from build123d import *
from build123d.topology import SkipClean

# Parameters (mm, degrees)
SKETCH_1_R               = 82.5
SKETCH_1_R_2             = 11.5
EXTRUDE_1_DEPTH          = 5
SKETCH_2_R               = 4
SKETCH_2_R_2             = 2.1
EXTRUDE_2_DEPTH          = 15
EXTRUDE_START            = 5
SKETCH_3_R               = 34
SKETCH_3_R_2             = 11.5
EXTRUDE_3_DEPTH          = 5
CUT_EXTRUDE_1_DEPTH      = 118.63290356
CUT_EXTRUDE_1_DEPTH_BACK = 10
SKETCH_4_R               = 82.5
EXTRUDE_4_DEPTH          = 5
SKETCH_6_R               = 11.5
CUT_EXTRUDE_2_DEPTH      = 109.80791311
SKETCH_7_R               = 34.75
SKETCH_7_R_2             = 11.5
EXTRUDE_5_DEPTH          = 5


with BuildPart() as part:
    # 草圖1 → 填料-伸長1 (new body)
    with BuildSketch(Plane(origin=(0, 0, 0), x_dir=(1, 0, 0), z_dir=(0, 1, 0))):
        with Locations(Location((0, 0, 0), (0, 0, 270))):
            Circle(SKETCH_1_R)
        with Locations(Location((0, 0, 0), (0, 0, 270))):
            Circle(SKETCH_1_R_2, mode=Mode.SUBTRACT)
    extrude(amount=EXTRUDE_1_DEPTH)

    # 草圖2 → 填料-伸長2 (add)
    # profile 1 of 3: a face of its own
    with BuildSketch(Plane(origin=(0, 5, 0), x_dir=(1, 0, 0), z_dir=(0, 1, 0))):
        with Locations(Location((0, 71.25, 0), (0, 0, 270))):
            Circle(SKETCH_2_R)
        with Locations(Location((0, 71.25, 0), (0, 0, 270))):
            Circle(SKETCH_2_R_2, mode=Mode.SUBTRACT)
    # profile 2 of 3: a face of its own
    with BuildSketch(Plane(origin=(0, 5, 0), x_dir=(1, 0, 0), z_dir=(0, 1, 0))):
        with Locations(Location((61.70431002, -35.625, 0), (0, 0, 270))):
            Circle(SKETCH_2_R)
        with Locations(Location((61.70431002, -35.625, 0), (0, 0, 270))):
            Circle(SKETCH_2_R_2, mode=Mode.SUBTRACT)
    # profile 3 of 3: a face of its own
    with BuildSketch(Plane(origin=(0, 5, 0), x_dir=(1, 0, 0), z_dir=(0, 1, 0))):
        with Locations(Location((-61.70431002, -35.625, 0), (0, 0, 270))):
            Circle(SKETCH_2_R)
        with Locations(Location((-61.70431002, -35.625, 0), (0, 0, 270))):
            Circle(SKETCH_2_R_2, mode=Mode.SUBTRACT)
    extrude(amount=EXTRUDE_2_DEPTH)

    # 草圖3 → 填料-伸長3 (add)
    with SkipClean():  # the faces are left unmerged after this step: merging them gives an invalid solid
        with BuildSketch(Plane.XZ.offset(EXTRUDE_START)):
            with Locations(Location((0, 0, 0), (0, 0, 90))):
                Circle(SKETCH_3_R)
            with Locations(Location((0, 0, 0), (0, 0, 270))):
                Circle(SKETCH_3_R_2, mode=Mode.SUBTRACT)
        extrude(amount=-EXTRUDE_3_DEPTH)

    # 草圖4 → 除料-伸長1 (cut, two sides: drawn at the far end of the back side and taken through both)
    with SkipClean():  # the faces are left unmerged after this step: merging them gives an invalid solid
        with BuildSketch(Plane(origin=(0, 5, 0), x_dir=(1, 0, 0), z_dir=(0, 1, 0)).offset(-CUT_EXTRUDE_1_DEPTH_BACK)):
            Circle(SKETCH_4_R)
            with BuildLine():
                ThreePointArc((-34.463200133, -38.269280586), (0, -51.5), (34.463200133, -38.269280586))
                ThreePointArc((34.463200133, -38.269280586), (40.109412614, -35.755030522), (46.155083654, -37.039954818))
                Line((46.155083654, -37.039954818), (57.20431002, -43.419228634))
                ThreePointArc((57.20431002, -43.419228634), (69.498538654, -40.125), (66.20431002, -27.830771366))
                Line((66.20431002, -27.830771366), (55.155083654, -21.451497549))
                ThreePointArc((55.155083654, -21.451497549), (51.019471053, -16.858254994), (50.373769239, -10.711366518))
                ThreePointArc((50.373769239, -10.711366518), (44.600308295, 25.75), (15.910569106, 48.980647104))
                ThreePointArc((15.910569106, 48.980647104), (10.910058438, 52.613285516), (9, 58.491452367))
                Line((9, 58.491452367), (9, 71.25))
                ThreePointArc((9, 71.25), (0, 80.25), (-9, 71.25))
                Line((-9, 71.25), (-9, 58.491452367))
                ThreePointArc((-9, 58.491452367), (-10.910058438, 52.613285516), (-15.910569106, 48.980647104))
                ThreePointArc((-15.910569106, 48.980647104), (-44.600308295, 25.75), (-50.373769239, -10.711366518))
                ThreePointArc((-50.373769239, -10.711366518), (-51.019471053, -16.858254994), (-55.155083654, -21.451497549))
                Line((-55.155083654, -21.451497549), (-66.20431002, -27.830771366))
                ThreePointArc((-66.20431002, -27.830771366), (-69.498538654, -40.125), (-57.20431002, -43.419228634))
                Line((-57.20431002, -43.419228634), (-46.155083654, -37.039954818))
                ThreePointArc((-46.155083654, -37.039954818), (-40.109412614, -35.755030522), (-34.463200133, -38.269280586))
            make_face(mode=Mode.SUBTRACT)
        extrude(amount=CUT_EXTRUDE_1_DEPTH + CUT_EXTRUDE_1_DEPTH_BACK, mode=Mode.SUBTRACT)

    # 草圖5 → 填料-伸長4 (add)
    with BuildSketch(Plane.XZ):
        with BuildLine():
            Line((-46.155083654, 37.039954818), (-57.20431002, 43.419228634))
            ThreePointArc((-57.20431002, 43.419228634), (-69.498538654, 40.125), (-66.20431002, 27.830771366))
            Line((-66.20431002, 27.830771366), (-55.155083654, 21.451497549))
            ThreePointArc((-55.155083654, 21.451497549), (-51.019471053, 16.858254994), (-50.373769239, 10.711366518))
            ThreePointArc((-50.373769239, 10.711366518), (-44.600308295, -25.75), (-15.910569106, -48.980647104))
            ThreePointArc((-15.910569106, -48.980647104), (-10.910058438, -52.613285516), (-9, -58.491452367))
            Line((-9, -58.491452367), (-9, -71.25))
            ThreePointArc((-9, -71.25), (0, -80.25), (9, -71.25))
            Line((9, -71.25), (9, -58.491452367))
            ThreePointArc((9, -58.491452367), (10.910058438, -52.613285516), (15.910569106, -48.980647104))
            ThreePointArc((15.910569106, -48.980647104), (44.600308295, -25.75), (50.373769239, 10.711366518))
            ThreePointArc((50.373769239, 10.711366518), (51.019471053, 16.858254994), (55.155083654, 21.451497549))
            Line((55.155083654, 21.451497549), (66.20431002, 27.830771366))
            ThreePointArc((66.20431002, 27.830771366), (69.498538654, 40.125), (57.20431002, 43.419228634))
            Line((57.20431002, 43.419228634), (46.155083654, 37.039954818))
            ThreePointArc((46.155083654, 37.039954818), (40.109412614, 35.755030522), (34.463200133, 38.269280586))
            ThreePointArc((34.463200133, 38.269280586), (0, 51.5), (-34.463200133, 38.269280586))
            ThreePointArc((-34.463200133, 38.269280586), (-40.109412614, 35.755030522), (-46.155083654, 37.039954818))
        make_face()
    extrude(amount=EXTRUDE_4_DEPTH)

    # 草圖6 → 除料-伸長2 (cut, through all)
    with BuildSketch(Plane(origin=(0, 0, 0), x_dir=(1, 0, 0), z_dir=(0, 1, 0))):
        with Locations(Location((0, 0, 0), (0, 0, 270))):
            Circle(SKETCH_6_R)
    extrude(amount=-CUT_EXTRUDE_2_DEPTH, mode=Mode.SUBTRACT)

    # 草圖7 → 填料-伸長5 (add)
    with SkipClean():  # the faces are left unmerged after this step: merging them gives an invalid solid
        with BuildSketch(Plane.XZ.offset(5)):
            with Locations(Location((0, 0, 0), (0, 0, 270))):
                Circle(SKETCH_7_R)
            with Locations(Location((0, 0, 0), (0, 0, 270))):
                Circle(SKETCH_7_R_2, mode=Mode.SUBTRACT)
        extrude(amount=EXTRUDE_5_DEPTH)
    add(part.part.scale(1), mode=Mode.REPLACE)  # the faces are merged on a copy


solid = part.part
For this review, take the finished solid that the model builds, in its own axes (mm). A direction names the side the tool comes from. Round coordinates to 2 decimals unless told otherwise and drop trailing zeros. Order: outer loops, then holes, each group sorted by start corner. A loop starts at its lowest first (then second) coordinate and runs counter-clockwise, first axis right, second up. Notation, with made-up numbers: (36, 74.5) -> (70, 74.5) arc R28 cw to (70, 106.5) -> close; hole circle Ø10 at (-33, 73). An arc over 180 degrees is marked (long way). Put each result on its own line as item: value.
Q1. Insertion check: pin 1 Ø5 at (x, z) = (0, -71.25) entering from +Y; pin 2 Ø1.3 at (x, z) = (-61.5, 36) entering from +Y; pin 3 Ø11 at (y, z) = (-0.5, -62) entering from -X; pin 4 Ø4 at (y, z) = (13, 31.5) entering from +X. Each pin has a flat end and moves straight along its axis. Give the tip position at first contact, or say it passes through.
Check result:
pin 1: y = 20
pin 2: y = 5
pin 3: x = -9.2
pin 4: x = 65.09
Q2. Machinability: for faces 1 (the flat face through (-27, -5, -24)), 2 (the flat face through (-9, 0, -65)), 3 (the flat face through (9, 0, -65)), which of the approach directions +Z, -Z, +X, -X, +Y, -Y give a long, thin tool a straight path to every point of the face, cutting with its end or side? Answer none if there is none.
Check result:
face 1: -Y
face 2: -Z, -X, +Y, -Y
face 3: -Z, +X, +Y, -Y
Q3. Add section B-B on x = 0. Write out the cut boundary in (y, z).
Check result:
outline: (-10, -34.75) -> (-5, -34.75) -> (-5, -80.25) -> (5, -80.25) -> (5, -75.25) -> (20, -75.25) -> (20, -73.35) -> (5, -73.35) -> (5, -69.15) -> (20, -69.15) -> (20, -67.25) -> (5, -67.25) -> (5, -11.5) -> (-10, -11.5) -> close; (-10, 11.5) -> (5, 11.5) -> (5, 51.5) -> (-5, 51.5) -> (-5, 34.75) -> (-10, 34.75) -> close
Q4. Mouldability with a two-part tool opening along Z and no side actions: class faces 4 (the flat face through (-51.602, 0.07, 40.185)), 5 (the cylindrical face through (0.176, 12.395, -75.246)), 6 (the flat face through (-62, 5, 36)) as pulls with the +Z half, pulls with the -Z half, needs draft (parallel to the pull), parting line crosses it, or undercut.
Check result:
face 4: pulls with the +Z half
face 5: parting line crosses it
face 6: undercut
Q5. Add section A-A on z = 0. Write out the cut boundary in (x, y), plus the area to 3 significant figures.
Check result:
outline: (-51.5, -5) -> (-34.75, -5) -> (-34.75, -10) -> (-11.5, -10) -> (-11.5, 5) -> (-51.5, 5) -> close; (11.5, -10) -> (34.75, -10) -> (34.75, -5) -> (51.5, -5) -> (51.5, 5) -> (11.5, 5) -> close
area: 1,030 mm2
Q6. Add section D-D on z = -26.5. Write out the cut boundary in (x, y).
Check result:
outline: (-44.16, -5) -> (-22.48, -5) -> (-22.48, -10) -> (22.48, -10) -> (22.48, -5) -> (44.16, -5) -> (44.16, 5) -> (-44.16, 5) -> close
Q7. For probe 1 along X at (y, z) = (-3.25, 0); probe 2 along Z at (x, y) = (0, 3.35); probe 3 along Y at (x, z) = (-23.5, 30.5), list the stretches that pass through material, from the lowest coordinate up. Write a range as [from, to].
Check result:
probe 1: [-51.5, -11.5], [11.5, 51.5]
probe 2: [-80.25, -11.5], [11.5, 51.5]
probe 3: [-5, 5]
Q8. Add section C-C on y = -8. Write out the cut boundary in (x, z).
Check result:
outline: circle Ø69.5 at (0, 0); hole circle Ø23 at (0, 0)
